Read the model definition and answer for the solid it produces. Units are mm, in the model's axes. A direction names the side the tool comes from. Coordinates: 2 decimals unless noted, no trailing zeros. Order: outer loops, then holes, each group sorted by start corner. A loop starts at its lowest first (then second) coordinate and runs counter-clockwise, first axis right, second up. Notation, with made-up numbers: M -14,-20.5 L -2,-20.5 A5 ccw -2,-12.5 Z; hole C 0,16.5 d9. An arc over 180 degrees is marked long. Write each question's results on one line, items separated by ' | '.
```python
from build123d import *

# Parameters (mm, degrees)
PAD_DEPTH       = 40
SKETCH001_R     = 2.25
SKETCH001_R_2   = 6
POCKET_DEPTH    = 1.601
COPYSKETCH002_R = 2.25
POCKET001_DEPTH = 5


with BuildPart() as part:
    # Sketch → Pad (new body)
    with BuildSketch(Plane.XZ):
        Polygon((0, 0), (0, 40), (1.6, 40), (1.6, 1.6), (40, 1.6), (40, 0), align=None)
    extrude(amount=PAD_DEPTH)

    # Sketch001 (on Face3 of Pad) → Pocket (cut, through all)
    with BuildSketch(Plane(origin=(1.6, 0, 0), x_dir=(0, 0, 1), z_dir=(1, 0, 0))):
        with Locations((10.6, 35)):
            Circle(SKETCH001_R)
        with Locations((31, 25)):
            Circle(SKETCH001_R)
        with Locations((10.6, 15)):
            Circle(SKETCH001_R)
        with Locations((31, 5)):
            Circle(SKETCH001_R)
        with Locations((20, 20)):
            Circle(SKETCH001_R_2)
    extrude(amount=-POCKET_DEPTH, mode=Mode.SUBTRACT)

    # CopySketch002 → Pocket001 (cut)
    with BuildSketch(Plane(origin=(0, 0, 2.5), x_dir=(-1, 0, 0), z_dir=(0, 0, 1))):
        with Locations((-11.5, 5)):
            Circle(COPYSKETCH002_R)
        with Locations((-31, 15)):
            Circle(COPYSKETCH002_R)
        with Locations((-11.5, 25)):
            Circle(COPYSKETCH002_R)
        with Locations((-31, 35)):
            Circle(COPYSKETCH002_R)
    extrude(amount=-POCKET001_DEPTH, mode=Mode.SUBTRACT)


solid = part.part
```
(1) The mould has two halves that part along Y. Classify faces 1 (the flat face through (11, -40, 1)), 2 (the flat face through (20, -20, 0)), 3 (the flat face through (11, 0, 1)), 4 (the cylindrical face through (29.962, -13.004, 0.811)): pulls with the +Y half, pulls with the -Y half, needs draft (parallel to the pull), parting line crosses it, or undercut.
Conclusion:
face 1: pulls with the -Y half | face 2: needs draft | face 3: pulls with the +Y half | face 4: undercut
(2) The part is cut by section A-A, the plane y = -5. Write down the section's boundary in (x, z), then the cut area to 3 significant figures.
Conclusion:
outline: M 0,0 L 9.25,0 L 9.25,1.6 L 1.6,1.6 L 1.6,28.75 L 0,28.75 Z; M 0,33.25 L 1.6,33.25 L 1.6,40 L 0,40 Z; M 13.75,0 L 40,0 L 40,1.6 L 13.75,1.6 Z | area: 111 mm²
(3) The part is cut by section C-C, the plane z = 10.6. Write down the section's boundary in (x, y).
Conclusion:
outline: M 0,-40 L 1.6,-40 L 1.6,-37.25 L 0,-37.25 Z; M 0,-32.75 L 1.6,-32.75 L 1.6,-17.25 L 0,-17.25 Z; M 0,-12.75 L 1.6,-12.75 L 1.6,0 L 0,0 Z
(4) The part is cut by section D-D, the plane y = -15. Write down the section's boundary in (x, z).
Conclusion:
outline: M 0,0 L 28.75,0 L 28.75,1.6 L 1.6,1.6 L 1.6,8.35 L 0,8.35 Z; M 0,12.85 L 1.6,12.85 L 1.6,16.68 L 0,16.68 Z; M 0,23.32 L 1.6,23.32 L 1.6,40 L 0,40 Z; M 33.25,0 L 40,0 L 40,1.6 L 33.25,1.6 Z
(5) For faces 5 (the cylindrical face through (0.811, -12.804, 10.112)), 6 (the flat face through (21, -20, 1.6)), determine the directions among +Z, -Z, +X, -X, +Y, -Y from which every point of the face is accessible in a straight line to the end or side of a thin tool.
Conclusion:
face 5: +X, -X | face 6: +Z, +X, +Y, -Y
(6) The part is cut by section B-B, the plane x = 31. Write down the section's boundary in (y, z).
Conclusion:
outline: M -40,0 L -37.25,0 L -37.25,1.6 L -40,1.6 Z; M -32.75,0 L -17.25,0 L -17.25,1.6 L -32.75,1.6 Z; M -12.75,0 L 0,0 L 0,1.6 L -12.75,1.6 Z
(7) Straight lines are drawn through the part: line 1 (Y direction, x = 0.4, z = 10.6); line 2 (Z direction, x = 0.4, y = -25); line 3 (Z direction, x = 3.5, y = -33). For each, find the intervals that lie inside material, in ascending order.
Conclusion:
line 1: -40 to -37.25, -32.75 to -17.25, -12.75 to 0 | line 2: 0 to 16.68, 23.32 to 28.75, 33.25 to 40 | line 3: 0 to 1.6
(8) Given pin 1 (4 mm diameter, centred on x = 11.5, y = -25, fed in from -Z); pin 2 (19 mm diameter, centred on y = -29, z = 30.5, fed in from +X); pin 3 (5 mm diameter, centred on x = 31, y = -35, fed in from +Z), each flat-ended and moving along its own axis, determine where each tip first touches the part or whether it passes through.
Conclusion:
pin 1: through | pin 2: x = 1.6 | pin 3: z = 1.6
